Design review of the part built by this model. Coordinates are the model's own, in mm. Face numbers are marked on the shaded views. A direction names the side the tool comes from. Round coordinates to 2 decimals unless told otherwise and drop trailing zeros. Order: outer loops, then holes, each group sorted by start corner. A loop starts at its lowest first (then second) coordinate and runs counter-clockwise, first axis right, second up. Notation, with made-up numbers: M 89,-1.75 L 113,-1.75 A16 ccw 113,17.25 Z; hole C 66,-39 d10. An arc over 180 degrees is marked long. Use a Markdown table: item, result. Add a question column.
(1) Machinability: for the marked faces 5, 6 and 7, which of the approach directions +Z, -Z, +X, -X, +Y, -Y give a long, thin tool a straight path to every point of the face, cutting with its end or side? Answer none if there is none.
(2) To check wall thickness, follow probe 1 along Y at (x, z) = (39, 48); probe 2 along X at (y, z) = (-25, -6); probe 3 along Z at (x, y) = (-3, -33). State the ranges of each line that lie inside material, in increasing order. Write a range as from..to.
(3) For pin 1 (1 mm diameter, centred on x = 6.5, y = -33.5, fed in from +Z); pin 2 (15 mm diameter, centred on x = 37.27, z = 26.79, fed in from -Y); pin 3 (1.5 mm diameter, centred on y = -43.5, z = 27.5, fed in from -X), all flat-tipped, find the tip position at first contact; note any pin that passes through.
(4) Take a section at D-D (z = 21). Write out the cut boundary in (x, y), then the cut area to 3 significant figures.
(5) The part is to be moulded in two halves that separate along X. For the marked faces 1, 2, 3 and 4, say which applies: released by +X, released by -X, zero draft, split by the parting line, or undercut.
(6) Take a section at A-A (z = 3). Write out the cut boundary in (x, y).
(7) Take a section at C-C (y = -17). Write out the cut boundary in (x, z).
(8) Take a section at B-B (x = 47.5). Write out the cut boundary in (y, z).
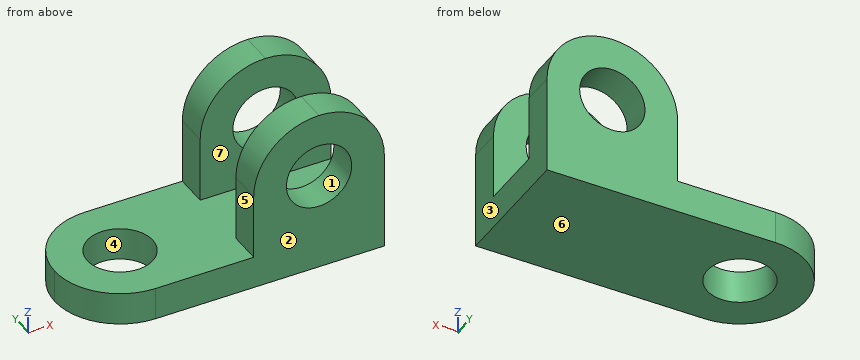
```python
from build123d import *

# Parameters (mm, degrees)
F0_W      = 114.3
F0_H      = 63.5
F1_DEPTH  = 50.8
F2_W      = 25.4
F2_H      = 57.0441053795
F3_DEPTH  = 114.301
F4_W      = 63.5
F4_H      = 12.7
F5_DEPTH  = 50.8
F6_W      = 63.5
F6_H      = 12.7
F7_DEPTH  = 50.8
F8_R      = 12.7
F9_DEPTH  = 50.801
F10_R     = 25.39999
F11_R     = 12.7
F12_DEPTH = 12.701


# Not quite as in the source:
# - a fillet or chamfer is up to 0.001 mm smaller than in the source, because OpenCascade refuses the exact size


with BuildPart() as f1:
    # F0 (on Front) → F1 (new body)
    with BuildSketch(Plane.XZ):
        with Locations((5.5195242167, 20.4444855223)):
            Rectangle(F0_W, F0_H)
    extrude(amount=F1_DEPTH)

    # F2 (on face) → F3 (cut, through all)
    with BuildSketch(Plane.YZ.offset(62.6695242167)):
        with Locations((-25.4, 29.9165382121)):
            Rectangle(F2_W, F2_H)
    extrude(amount=-F3_DEPTH, mode=Mode.SUBTRACT)

    # F4 (on face) → F5 (cut)
    with BuildSketch(Plane.XY.offset(52.1944855223)):
        with Locations((-19.8804757833, -44.45)):
            Rectangle(F4_W, F4_H)
    extrude(amount=-F5_DEPTH, mode=Mode.SUBTRACT)

    # F6 (on face) → F7 (cut)
    with BuildSketch(Plane.XY.offset(52.1944855223)):
        with Locations((-19.8804757833, -6.35)):
            Rectangle(F6_W, F6_H)
    extrude(amount=-F7_DEPTH, mode=Mode.SUBTRACT)

    # F8 (on face) → F9 (cut, through all)
    with BuildSketch(Plane.XZ.offset(50.8)):
        with Locations((37.2695242167, 26.7944855223)):
            Circle(F8_R)
    extrude(amount=-F9_DEPTH, mode=Mode.SUBTRACT)

    # F10 (radius 25.4 in the source; OpenCascade refuses exactly that, so slightly less here)
    f10_edges = [f1.edges().sort_by_distance(p)[0] for p in [
        (62.669524, -44.45, 52.194486),
        (11.869524, -44.45, 52.194486),
        (11.869524, -6.35, 52.194486),
        (62.669524, -6.35, 52.194486),
        (-51.630476, -50.8, -4.955514),
        (-51.630476, 0, -4.955514),
    ]]
    fillet(f10_edges, radius=F10_R)

    # F11 (on face) → F12 (cut, through all)
    with BuildSketch(Plane.XY.offset(1.3944855223)):
        with Locations((-26.2304757833, -25.4)):
            Circle(F11_R)
    extrude(amount=-F12_DEPTH, mode=Mode.SUBTRACT)


solid = f1.part
```
Verdict:
| question | item | result |
|---|---|---|
| 1 | face 5 | +Z, -X, +Y, -Y |
| 1 | face 6 | -Z, +X, -X, +Y, -Y |
| 1 | face 7 | +Z, +X, -X |
| 2 | probe 1 | y = -50.8..-38.1, -12.7..0 |
| 2 | probe 2 | x = -51.63..-38.92, -13.54..62.67 |
| 2 | probe 3 | z = -11.31..1.39 |
| 3 | pin 1 | stops at z = 1.39 |
| 3 | pin 2 | passes through |
| 3 | pin 3 | stops at x = 11.87 |
| 4 | outline | M 11.87,-50.8 L 25.97,-50.8 L 25.97,-38.1 L 11.87,-38.1 Z; M 11.87,-12.7 L 25.97,-12.7 L 25.97,0 L 11.87,0 Z; M 48.57,-50.8 L 62.67,-50.8 L 62.67,-38.1 L 48.57,-38.1 Z; M 48.57,-12.7 L 62.67,-12.7 L 62.67,0 L 48.57,0 Z |
| 4 | area | 716 mm^2 |
| 5 | face 1 | undercut |
| 5 | face 2 | zero draft |
| 5 | face 3 | released by +X |
| 5 | face 4 | undercut |
| 6 | outline | M 11.87,-50.8 L 62.67,-50.8 L 62.67,-38.1 L 11.87,-38.1 Z; M 11.87,-12.7 L 62.67,-12.7 L 62.67,0 L 11.87,0 Z |
| 7 | outline | M -50.2,-11.31 L -35.76,-11.31 L -35.76,1.39 L -50.2,1.39 Z; M -16.71,-11.31 L 62.67,-11.31 L 62.67,1.39 L -16.71,1.39 Z |
| 8 | outline | M -50.8,-11.31 L 0,-11.31 L 0,19.27 L -12.7,19.27 L -12.7,1.39 L -38.1,1.39 L -38.1,19.27 L -50.8,19.27 Z; M -50.8,34.32 L -38.1,34.32 L -38.1,50.04 L -50.8,50.04 Z; M -12.7,34.32 L 0,34.32 L 0,50.04 L -12.7,50.04 Z |
